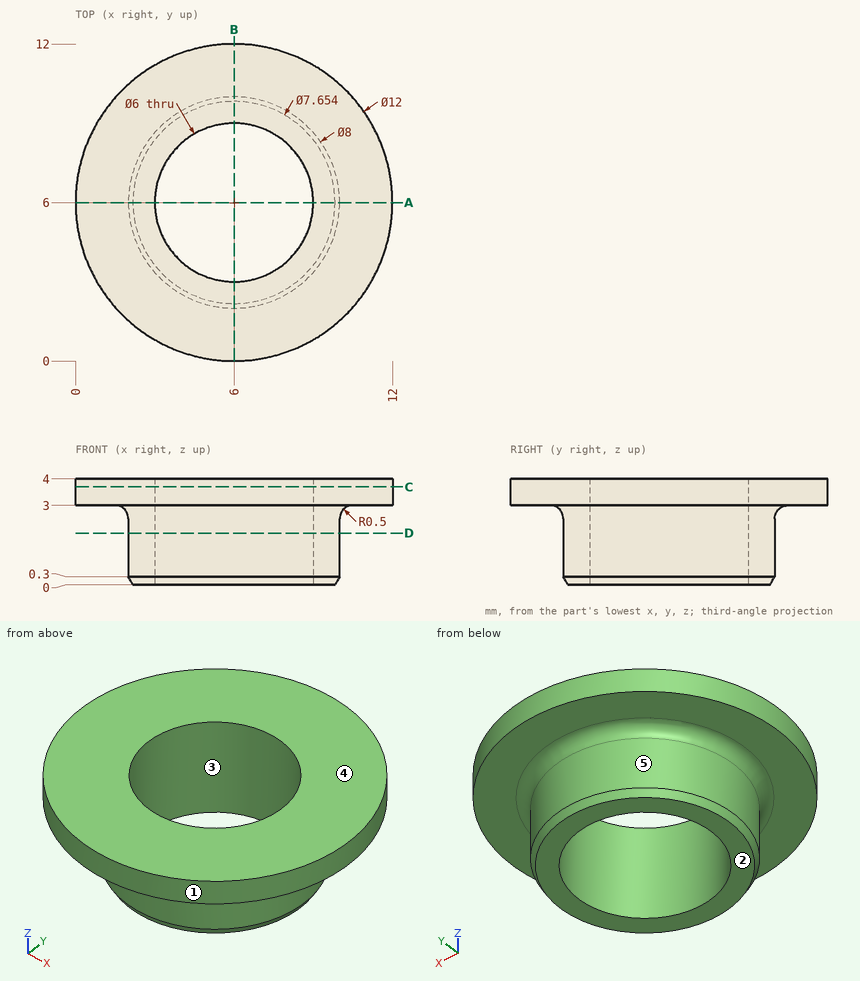
Study the drawing (mm; zero at the part's minimum x, y, z) and answer. A direction names the side the tool comes from. Give positions to 0.01 mm unless a question says otherwise; leave off trailing zeros. Loops run counter-clockwise (first coordinate to the right, second up) from the corner with the lowest first, then second, coordinate; pieces in that order, holes last. Notation, with made-up numbers: (84, 84.25) - (131, 84.25) arc R26 cw to (131, 99.25) - close; hole circle Ø9 at (4.5, 74.25). An arc over 180 degrees is marked (long way). Answer in a Markdown table with one row per item. Add a question column.
Q1. A tool of negligible diameter and unlimited length cuts with its end or side. For the marked faces 4 and 5, from which of +Z, -Z, +X, -X, +Y, -Y can it reach the whole face along a straight path? Write none if from no direction.
Q2. Each of these flat-tipped pins is pushed along its axis until it touches: P1, Ø1.5, axis at y = 2.5, z = 1, coming from the +X side (1 decimal); P2, Ø1.5, axis at y = 7, z = 2.5, coming from the -X side; P3, Ø1.5, axis at x = 3, z = 3, coming from the -Y side. Where does it stop, or does it pass through?
Q3. The part is cut by section C-C (z = 3.7). Determine the outline of the cut face in (x, y).
Q4. Consider line 1 along Y through (x, z) = (6, 1.55); line 2 along Y through (x, z) = (5, 0.7); line 3 along Z through (x, y) = (4.5, 1). Determine where each line is inside the solid, lowest interval first.
Q5. The part is cut by section A-A (y = 6). Determine the outline of the cut face in (x, z).
Q6. Determine the mould class of the marked faces 1, 2 and 3 for opening direction Y: released by +Y, released by -Y, zero draft, split by the parting line, or undercut.
Q7. The part is cut by section D-D (z = 1.95). Determine the outline of the cut face in (x, y).
Solution:
| question | item | result |
|---|---|---|
| 1 | face 4 | +Z, +X, -X, +Y, -Y |
| 1 | face 5 | -Z |
| 2 | P1 | stops at x = 8.9 |
| 2 | P2 | stops at x = 0.02 |
| 2 | P3 | stops at y = 0.44 |
| 3 | outline | circle Ø12 at (6, 6); hole circle Ø6 at (6, 6) |
| 4 | line 1 | y = 2 to 3, 9 to 10 |
| 4 | line 2 | y = 2.13 to 3.17, 8.83 to 9.87 |
| 4 | line 3 | z = 3 to 4 |
| 5 | outline | (0, 3) - (1.5, 3) arc R0.5 cw to (2, 2.5) - (2, 0.3) - (2.17, 0) - (3, 0) - (3, 4) - (0, 4) - close; (9, 0) - (9.83, 0) - (10, 0.3) - (10, 2.5) arc R0.5 cw to (10.5, 3) - (12, 3) - (12, 4) - (9, 4) - close |
| 6 | face 1 | split by the parting line |
| 6 | face 2 | zero draft |
| 6 | face 3 | undercut |
| 7 | outline | circle Ø8 at (6, 6); hole circle Ø6 at (6, 6) |
